Autodesk Inventor part; units mm, degrees
ref_plane "YZ Plane" through (0, 0, 0) normal (1, 0, 0) x (0, 1, 0)
ref_plane "XZ Plane" through (0, 0, 0) normal (0, 1, 0) x (-1, 0, 0)
ref_plane "XY Plane" through (0, 0, 0) normal (0, 0, 1) x (1, 0, 0)
sketch "Skizze1" plane through (0, 0, 0) normal (0, 0, 1) x (1, 0, 0)
  line L0 (-2.9798, 1.7507) -> (0.0263, 3.4559)
  line L1 (0.0263, 3.4559) -> (3.0061, 1.7052)
  line L2 (3.0061, 1.7052) -> (2.9798, -1.7507)
  line L3 (2.9798, -1.7507) -> (-0.0263, -3.4559)
  line L4 (-0.0263, -3.4559) -> (-3.0061, -1.7052)
  line L5 (-3.0061, -1.7052) -> (-2.9798, 1.7507)
  point P0 (0, 0)
extrude "Extrusion1" add sketch "Skizze1" along normal blind 2.4
sketch "Skizze2" plane through (0, 0, 2.4) normal (0, 0, 1) x (1, 0, 0)
  circle A0 centre (0, 0) radius 1.5
  dimension "d3" = 3
extrude "Extrusion2" cut sketch "Skizze2" against normal through all
thread "Gewinde1"
properties part number "M3 Mutter"
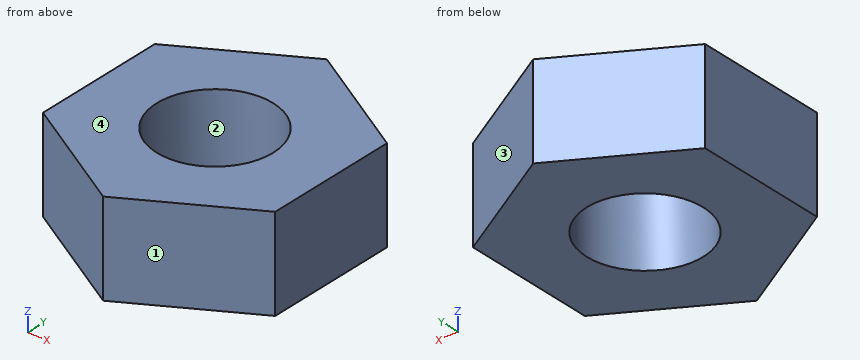
Design review of the part built by this model. Coordinates are the model's own, in mm. Face numbers are marked on the shaded views. Coordinates: 2 decimals unless noted, no trailing zeros. Order: outer loops, then holes, each group sorted by start corner. A loop starts at its lowest first (then second) coordinate and runs counter-clockwise, first axis right, second up. Notation, with made-up numbers: (24.5, 32) - (71.5, 32) arc R32 ccw to (71.5, 65) - close; hole circle Ø3 at (-37, 71.25). An arc over 180 degrees is marked (long way). Answer in a Markdown table with one row per item.
(1) Wall thickness on line 1 along X through (y, z) = (1.25, 1.4); line 2 along Y through (x, z) = (0.5, 2.35); line 3 along Y through (x, z) = (0, 0.8): over which ranges is each line inside the solid? List them lowest first. Write a range as from..to.
Checked values:
| item | result |
|---|---|
| line 1 | -2.98..-0.83, 0.83..3 |
| line 2 | -3.16..-1.41, 1.41..3.18 |
| line 3 | -3.44..-1.5, 1.5..3.44 |
(2) Consider section A-A on y = 0. State the section outline as (x, z) points.
Checked values:
| item | result |
|---|---|
| outline | (-2.99, 0) - (-1.5, 0) - (-1.5, 2.4) - (-2.99, 2.4) - close; (1.5, 0) - (2.99, 0) - (2.99, 2.4) - (1.5, 2.4) - close |
(3) The part is to be moulded in two halves that separate along Y. For the marked faces 1, 2, 3 and 4, say which applies: released by +Y, released by -Y, zero draft, split by the parting line, or undercut.
Checked values:
| item | result |
|---|---|
| face 1 | released by -Y |
| face 2 | undercut |
| face 3 | released by +Y |
| face 4 | zero draft |
(4) Consider section C-C on x = -0.25. State the section outline as (y, z) points.
Checked values:
| item | result |
|---|---|
| outline | (-3.32, 0) - (-1.48, 0) - (-1.48, 2.4) - (-3.32, 2.4) - close; (1.48, 0) - (3.3, 0) - (3.3, 2.4) - (1.48, 2.4) - close |
(5) Consider section B-B on z = 0.95. State the section outline as (x, y) points, plus the area to 3 significant figures.
Checked values:
| item | result |
|---|---|
| outline | (-3.01, -1.71) - (-0.03, -3.46) - (2.98, -1.75) - (3.01, 1.71) - (0.03, 3.46) - (-2.98, 1.75) - close; hole circle Ø3 at (0, 0) |
| area | 24.0 mm^2 |
(6) Consider section D-D on x = 1.75. State the section outline as (y, z) points, plus the area to 3 significant figures.
Checked values:
| item | result |
|---|---|
| outline | (-2.45, 0) - (2.44, 0) - (2.44, 2.4) - (-2.45, 2.4) - close |
| area | 11.7 mm^2 |
